Source: CAD feature listing. Evaluate the final solid. Frame: model axes, mm. Round coordinates to 2 decimals unless told otherwise and drop trailing zeros. Loops run counter-clockwise (first coordinate to the right, second up) from the corner with the lowest first, then second, coordinate; pieces in that order, holes last.
(1) First-contact query: pin 1 Ø2 at (x, z) = (35, 1.5) entering from +Y. Flat tip, straight axial feed; report the tip coordinate or a pass-through.
(2) Section D-D, the plane x = 35. Return the cut outline in (y, z), plus the area to 3 significant figures.
(3) Section B-B, the plane z = 0.7. Count the separate pieces of the cut face and the enclosed holes in it, plus the area to 3 significant figures.
(4) Section C-C, the plane x = -19. Return the cut outline in (y, z), plus the area to 3 significant figures.
(5) Material intervals for probe 1 along X at (y, z) = (7, 0.85); probe 2 along Y at (x, z) = (17.5, 1.7); probe 3 along X at (y, z) = (60, 0.85), sorted ascending.
(6) Section A-A, the plane y = 31.5. Return the cut outline in (x, z).
```python
from build123d import *

# Parameters (mm, degrees)
F0_W        = 7
F0_H        = 5
F1_DEPTH    = 4
F2_T1_DEPTH = 4
F2_T3_DEPTH = 14
F2_T5_DEPTH = 5.7632698071


# Not quite as in the source:
# - a fillet or chamfer that OpenCascade refuses, or shapes differently, is made with other operations: its cross-section is extruded or revolved along the edge and cut away or added


with BuildPart() as f1:
    # F0 (on Top) → F1 (new body)
    with BuildSketch(Plane.XY):
        with BuildLine():
            Line((-51, -4), (44, -4))
            Line((44, -4), (44, 0))
            Line((44, 0), (40.8074666826, 0))
            Line((40.8074666826, 0), (29.3850666349, 0))
            Line((29.3850666349, 0), (26.1925333174, 0))
            Line((26.1925333174, 0), (14.6925333174, 0))
            Line((14.6925333174, 0), (11.5, 0))
            Line((11.5, 0), (0, 0))
            Line((0, 0), (-44.4302483166, 139.9080159757))
            ThreePointArc((-44.4302483166, 139.9080159757), (-45.5180993372, 141.4211616971), (-47.2895326655, 142))
            Line((-47.2895326655, 142), (-48, 142))
            ThreePointArc((-48, 142), (-50.1213203436, 141.1213203436), (-51, 139))
            Line((-51, 139), (-51, -4))
        make_face()
        with Locations((-40.5, 2.5)):
            Rectangle(F0_W, F0_H, mode=Mode.SUBTRACT)
        with Locations((-26.5, 2.5)):
            Rectangle(F0_W, F0_H, mode=Mode.SUBTRACT)
        with Locations((-12.5, 2.5)):
            Rectangle(F0_W, F0_H, mode=Mode.SUBTRACT)
        with BuildLine():
            Line((-7.3725300405, 9), (-47, 9))
            ThreePointArc((-47, 9), (-47.7071067812, 9.2928932188), (-48, 10))
            Line((-48, 10), (-48, 71.4074290533))
            ThreePointArc((-48, 71.4074290533), (-47.7071067812, 72.1145358345), (-47, 72.4074290533))
            Line((-47, 72.4074290533), (-26.8735379155, 72.4074290533))
            ThreePointArc((-26.8735379155, 72.4074290533), (-26.2830601394, 72.2144829523), (-25.9204431326, 71.7101010452))
            Line((-25.9204431326, 71.7101010452), (-6.4194352575, 10.3026719919))
            ThreePointArc((-6.4194352575, 10.3026719919), (-6.5654761415, 9.4095222239), (-7.3725300405, 9))
        make_face(mode=Mode.SUBTRACT)
        with Locations((-37.5, 76.9074290533)):
            Rectangle(F0_W, F0_H, mode=Mode.SUBTRACT)
        with BuildLine():
            ThreePointArc((-48, 134.7843734895), (-47.1531424452, 135.7725776139), (-46.046905217, 135.0870454814))
            Line((-46.046905217, 135.0870454814), (-29.4136863758, 82.7101010452))
            ThreePointArc((-29.4136863758, 82.7101010452), (-29.5597272597, 81.8169512772), (-30.3667811588, 81.4074290533))
            Line((-30.3667811588, 81.4074290533), (-47, 81.4074290533))
            ThreePointArc((-47, 81.4074290533), (-47.7071067812, 81.7003222721), (-48, 82.4074290533))
            Line((-48, 82.4074290533), (-48, 134.7843734895))
        make_face(mode=Mode.SUBTRACT)
        Polygon((40.8074666826, 0), (44, 0), (40.2063431117, 10.4229866378), (37.3872652493, 9.3969262079), align=None)
        Polygon((26.1925333174, 0), (29.3850666349, 0), (25.5914097465, 10.4229866378), (22.7723318842, 9.3969262079), align=None)
        Polygon((11.5, 0), (14.6925333174, 0), (10.8988764291, 10.4229866378), (8.0797985667, 9.3969262079), align=None)
    extrude(amount=F1_DEPTH)

    # F2: fillet of radius 2 on 15 edges, made by hand

    # F2_s2 → F2_t1 (join)
    with BuildSketch(Plane.XY):
        with BuildLine():
            ThreePointArc((39.8305559107, 2.6840402867), (39.5894747577, 0.8528471273), (37.9511706691, 0))
            Line((37.9511706691, 0), (40.8074666826, 0))
            Line((40.8074666826, 0), (39.8305559107, 2.6840402867))
        make_face()
        with BuildLine():
            ThreePointArc((16.0929483938, 0), (14.9457955211, 0.3616959114), (14.2135631523, 1.3159597133))
            Line((14.2135631523, 1.3159597133), (14.6925333174, 0))
            Line((14.6925333174, 0), (16.0929483938, 0))
        make_face()
        with BuildLine():
            ThreePointArc((10.5230892281, 2.6840402867), (10.2820080751, 0.8528471273), (8.6437039865, 0))
            Line((8.6437039865, 0), (11.5, 0))
            Line((11.5, 0), (10.5230892281, 2.6840402867))
        make_face()
        with BuildLine():
            ThreePointArc((1.4632920473, 0), (0.2823364951, 0.3858922019), (-0.4428975187, 1.3946560162))
            Line((-0.4428975187, 1.3946560162), (0, 0))
            Line((0, 0), (1.4632920473, 0))
        make_face()
        with BuildLine():
            ThreePointArc((25.2156225455, 2.6840402867), (24.9745413925, 0.8528471273), (23.3362373039, 0))
            Line((23.3362373039, 0), (26.1925333174, 0))
            Line((26.1925333174, 0), (25.2156225455, 2.6840402867))
        make_face()
        with BuildLine():
            ThreePointArc((30.7854817113, 0), (29.6383288386, 0.3616959114), (28.9060964697, 1.3159597133))
            Line((28.9060964697, 1.3159597133), (29.3850666349, 0))
            Line((29.3850666349, 0), (30.7854817113, 0))
        make_face()
    extrude(amount=F2_T1_DEPTH)

    # F2_s4 → F2_t3 (cut)
    with BuildSketch(Plane.XY.offset(-5)):
        with BuildLine():
            ThreePointArc((-51, -2), (-50.4142135624, -3.4142135624), (-49, -4))
            Line((-49, -4), (-51, -4))
            Line((-51, -4), (-51, -2))
        make_face()
        with BuildLine():
            ThreePointArc((42, -4), (43.4142135624, -3.4142135624), (44, -2))
            Line((44, -2), (44, -4))
            Line((44, -4), (42, -4))
        make_face()
        with BuildLine():
            ThreePointArc((40.8903833983, 8.5436013963), (39.8562346802, 9.6721766837), (38.3269578701, 9.7389463512))
            Line((38.3269578701, 9.7389463512), (40.2063431117, 10.4229866378))
            Line((40.2063431117, 10.4229866378), (40.8903833983, 8.5436013963))
        make_face()
        with BuildLine():
            ThreePointArc((39.2666504909, 10.0809664945), (38.1380752035, 9.0468177764), (38.071305536, 7.5175409663))
            Line((38.071305536, 7.5175409663), (37.3872652493, 9.3969262079))
            Line((37.3872652493, 9.3969262079), (39.2666504909, 10.0809664945))
        make_face()
        with BuildLine():
            ThreePointArc((11.5829167158, 8.5436013963), (10.5487679977, 9.6721766837), (9.0194911875, 9.7389463512))
            Line((9.0194911875, 9.7389463512), (10.8988764291, 10.4229866378))
            Line((10.8988764291, 10.4229866378), (11.5829167158, 8.5436013963))
        make_face()
        with BuildLine():
            ThreePointArc((9.9591838083, 10.0809664945), (8.8306085209, 9.0468177764), (8.7638388534, 7.5175409663))
            Line((8.7638388534, 7.5175409663), (8.0797985667, 9.3969262079))
            Line((8.0797985667, 9.3969262079), (9.9591838083, 10.0809664945))
        make_face()
        with BuildLine():
            ThreePointArc((24.6517171257, 10.0809664945), (23.5231418383, 9.0468177764), (23.4563721708, 7.5175409663))
            Line((23.4563721708, 7.5175409663), (22.7723318842, 9.3969262079))
            Line((22.7723318842, 9.3969262079), (24.6517171257, 10.0809664945))
        make_face()
        with BuildLine():
            ThreePointArc((26.2754500332, 8.5436013963), (25.2413013151, 9.6721766837), (23.712024505, 9.7389463512))
            Line((23.712024505, 9.7389463512), (25.5914097465, 10.4229866378))
            Line((25.5914097465, 10.4229866378), (26.2754500332, 8.5436013963))
        make_face()
    extrude(amount=F2_T3_DEPTH, mode=Mode.SUBTRACT)

    # F2_s6 → F2_t5 (cut)
    with BuildSketch(Plane.XY.offset(-0.8816349035)):
        with BuildLine():
            ThreePointArc((44, -0.3526539614), (43.969615506, -0.0053576061), (43.8793852416, 0.3313863252))
            Line((43.8793852416, 0.3313863252), (44, 0))
            Line((44, 0), (44, -0.3526539614))
        make_face()
    extrude(amount=F2_T5_DEPTH, mode=Mode.SUBTRACT)


solid = f1.part
```
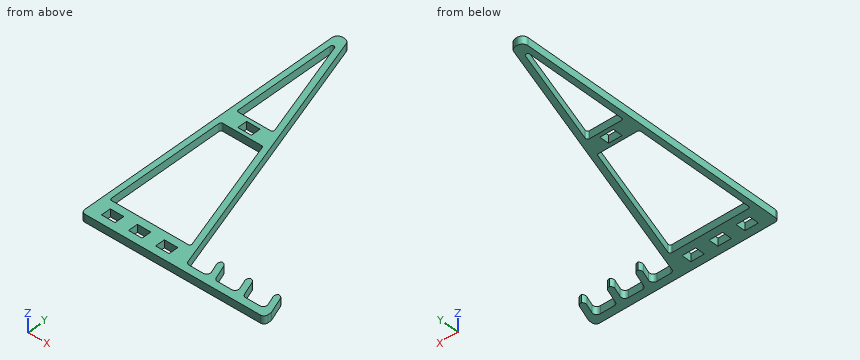
Output values:
1. pin 1: stops at y = 0
2. outline: (-4, 0) - (0, 0) - (0, 4) - (-4, 4) - close
2. area: 16.0 mm2
3. separate pieces: 1
3. enclosed holes: 6
3. area: 1,790 mm2
4. outline: (-4, 0) - (9, 0) - (9, 4) - (-4, 4) - close; (49.92, 0) - (59.83, 0) - (59.83, 4) - (49.92, 4) - close
4. area: 91.6 mm2
5. probe 1: x = -51 to -2.22, 8.95 to 12.14, 23.64 to 26.84, 38.26 to 41.45
5. probe 2: y = -4 to 0
5. probe 3: x = -51 to -48, -22.2 to -19.05
6. outline: (-51, 0) - (-48, 0) - (-48, 4) - (-51, 4) - close; (-13.15, 0) - (-10, 0) - (-10, 4) - (-13.15, 4) - close
